```python
from build123d import *

# Parameters (mm, degrees)
F0_W     = 127
F0_H     = 127
F1_DEPTH = 127


with BuildPart() as f1:
    # F0 (on Top) → F1 (new body)
    with BuildSketch(Plane.XY):
        Polygon((-127, 0), (0, 0), (0, 127), (0, 254), (0, 381), (0, 508), (0, 635), (-127, 635), (-254, 635), (-381, 635), (-508, 635), (-635, 635), (-635, 508), (-635, 381), (-635, 254), (-635, 127), (-635, 0), (-508, 0), (-381, 0), (-254, 0), align=None)
        with Locations((-190.5, -63.5)):
            Rectangle(F0_W, F0_H)
        with Locations((63.5, 190.5)):
            Rectangle(F0_W, F0_H)
        with Locations((-444.5, -63.5)):
            Rectangle(F0_W, F0_H)
        with Locations((63.5, 444.5)):
            Rectangle(F0_W, F0_H)
        with Locations((-698.5, 190.5)):
            Rectangle(F0_W, F0_H)
        with Locations((-190.5, 698.5)):
            Rectangle(F0_W, F0_H)
        with Locations((-698.5, 444.5)):
            Rectangle(F0_W, F0_H)
        with Locations((-444.5, 698.5)):
            Rectangle(F0_W, F0_H)
    extrude(amount=F1_DEPTH)


solid = f1.part
```
Input: part model. Units: mm. Frame: model coordinates. A direction names the side the tool comes from. Give positions to 0.01 mm unless a question says otherwise; leave off trailing zeros. Order: outer loops, then holes, each group sorted by start corner. A loop starts at its lowest first (then second) coordinate and runs counter-clockwise, first axis right, second up. Notation, with made-up numbers: M 36,67.5 L 54,67.5 A12 cw 54,89.5 Z; hole C 16,33 d7. An arc over 180 degrees is marked long. Return JSON: item names as keys, results as strings.
1) Line query: L1, parallel to Y at x = 42, z = 108; L2, parallel to X at y = 299.5, z = 100.5; L3, parallel to Y at x = -114.5, z = 45. Output: solid intervals per line, ascending. Write a range as [from, to].
Taken from the geometry:
{"L1": "y = [127, 254], [381, 508]", "L2": "x = [-635, 0]", "L3": "y = [0, 635]"}
2) Mould query, pull axis Y, two halves, no side actions, for faces 1 (the face through (63, 254, 63)), 2 (the face through (-699, 508, 63)), 3 (the face through (-635, 64, 63)). Classes: released by +Y, released by -Y, zero draft, split by the parting line, or undercut.
Taken from the geometry:
{"face 1": "undercut", "face 2": "released by +Y", "face 3": "zero draft"}
3) Contact query for flat-ended pins moving along their axis: pin 1 (1 mm diameter, centred on y = 673, z = 40, fed in from -X); pin 2 (2 mm diameter, centred on x = -641, z = 48.5, fed in from +Y); pin 3 (4 mm diameter, centred on x = -148, y = 489.5, fed in from -Z); pin 4 (1 mm diameter, centred on x = -346, z = 101.5, fed in from -Y). Output: stop coordinate, or through.
Taken from the geometry:
{"pin 1": "stops at x = -508", "pin 2": "stops at y = 508", "pin 3": "stops at z = 0", "pin 4": "stops at y = 0"}
4) Section query A-A on y = -64. Output: boundary loops of the cut face in (x, z), and give its area (3 significant figures).
Taken from the geometry:
{"outline": "M -508,0 L -381,0 L -381,127 L -508,127 Z; M -254,0 L -127,0 L -127,127 L -254,127 Z", "area": "32,300 mm2"}
5) Section query C-C on y = 292. Output: boundary loops of the cut face in (x, z), and give its area (3 significant figures).
Taken from the geometry:
{"outline": "M -635,0 L 0,0 L 0,127 L -635,127 Z", "area": "80,600 mm2"}
6) Access query for faces 4 (the face through (-635, 318, 63)), 5 (the face through (-381, 698, 63)), 6 (the face through (-572, 0, 63)), 7 (the face through (-381, -64, 63)). Directions: +Z, -Z, +X, -X, +Y, -Y. A direction counts if a zero-diameter tool reaches every point of the face in a straight line with its end or side. Return the directions, or none.
Taken from the geometry:
{"face 4": "+Z, -Z, -X", "face 5": "+Z, -Z, +Y", "face 6": "+Z, -Z, -X, -Y", "face 7": "+Z, -Z, -Y"}
7) Section query B-B on x = -647. Output: boundary loops of the cut face in (y, z).
Taken from the geometry:
{"outline": "M 127,0 L 254,0 L 254,127 L 127,127 Z; M 381,0 L 508,0 L 508,127 L 381,127 Z"}
